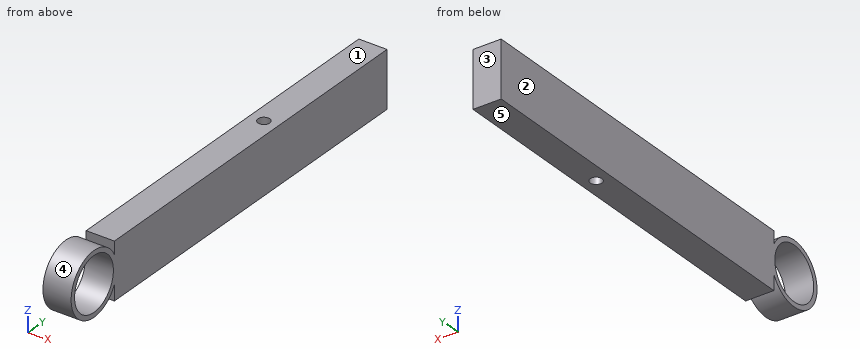
```python
from build123d import *

# Parameters (mm, degrees)
F0_W     = 19.05
F0_H     = 38.1
F1_DEPTH = 127
F2_R     = 18.0975
F3_DEPTH = 19.05
F5_R     = 3.96875
F6_DEPTH = 39.371


with BuildPart() as f1:
    # F0 (on Front) → F1 (new body, symmetric)
    with BuildSketch(Plane.XZ):
        with Locations((9.525, 19.05)):
            Rectangle(F0_W, F0_H)
    extrude(amount=F1_DEPTH, both=True)


with BuildPart() as f3:
    # F2 (on face) → F3 (new body)
    with BuildSketch(Plane.YZ.offset(19.05)):
        with BuildLine():
            Line((-127, 10.535887), (-127, 29.469113))
            ThreePointArc((-127, 29.469113), (-167.3225, 20.0025), (-127, 10.535887))
        make_face()
        with Locations((-146.05, 20.0025)):
            Circle(F2_R, mode=Mode.SUBTRACT)
    extrude(amount=-F3_DEPTH)

    # F4: union F1
    add(f1.part)

    # F5 (on face) → F6 (cut, through all)
    with BuildSketch(Plane.XY.offset(38.1)):
        with Locations((9.525, 25.4)):
            Circle(F5_R)
    extrude(amount=-F6_DEPTH, mode=Mode.SUBTRACT)


solid = f3.part
```
Read the model definition and answer for the solid it produces. Units are mm, in the model's axes. Face numbers are marked on the shaded views. A direction names the side the tool comes from. Give positions to 0.01 mm unless a question says otherwise; leave off trailing zeros. Loops run counter-clockwise (first coordinate to the right, second up) from the corner with the lowest first, then second, coordinate; pieces in that order, holes last.
Item 1: For the marked faces 1 and 2, determine the directions among +Z, -Z, +X, -X, +Y, -Y from which every point of the face is accessible in a straight line to the end or side of a thin tool.
Item 2: Each of these flat-tipped pins is pushed along its axis until it touches: pin 1 Ø9.5 at (x, z) = (9, 32.5) entering from -Y; pin 2 Ø3 at (x, z) = (12.5, 3.5) entering from -Y; pin 3 Ø2 at (x, y) = (9, 63.5) entering from -Z. Where does it stop, or does it pass through?
Item 3: The mould has two halves that part along Y. Classify the marked faces 3, 4 and 5: released by +Y, released by -Y, zero draft, split by the parting line, or undercut.
Item 4: Find the intervals of material crossed by line 1 along X through (y, z) = (25, 1.5); line 2 along Y through (x, z) = (3, 21); line 3 along Z through (x, y) = (5.75, -146.05) (3 decimals), in increasing order.
Item 5: The part is cut by section B-B (z = 35.5). Give the number of separate pieces and of enclosed holes in the cut face, and give its area (3 significant figures).
Item 6: The part is cut by section A-A (y = -146.05). Write down the section's boundary in (x, z) (3 decimals), and give its area (3 significant figures).
Taken from the geometry:
1. face 1: +Z, +X, -X, +Y
1. face 2: +Z, -Z, -X, +Y, -Y
2. pin 1: stops at y = -165.86
2. pin 2: stops at y = -161.13
2. pin 3: stops at z = 0
3. face 3: released by +Y
3. face 4: undercut
3. face 5: zero draft
4. line 1: x = 0 to 5.58, 13.47 to 19.05
4. line 2: y = -167.3 to -164.12, -127.98 to 127
4. line 3: z = -1.27 to 1.905, 38.1 to 41.275
5. separate pieces: 3
5. enclosed holes: 1
5. area: 4,990 mm2
6. outline: (0, -1.27) - (19.05, -1.27) - (19.05, 1.905) - (0, 1.905) - close; (0, 38.1) - (19.05, 38.1) - (19.05, 41.275) - (0, 41.275) - close
6. area: 121 mm2
